from build123d import *

# Parameters (mm, degrees)
F0_R     = 6.35
F1_DEPTH = 25.4
F3_DEPTH = 12.7
F4_W     = 6.35
F4_H     = 114.3
F5_DEPTH = 25.4


with BuildPart() as f1:
    # F0 (on Front) → F1 (new body)
    with BuildSketch(Plane.XZ):
        with Locations((3.9284797385, 25.3006741405)):
            Circle(F0_R)
    extrude(amount=F1_DEPTH)



with BuildPart() as f1b:
    # F0 (on Front) → F1, piece 2 (new body)
    with BuildSketch(Plane.XZ):
        with Locations((3.9284797385, -177.8993258595)):
            Circle(F0_R)
    extrude(amount=F1_DEPTH)


with BuildPart() as f1_1:
    add(f1.part)

    add(f1b.part)  # F3 merges F1b
    # F2 (on face) → F3 (join)
    with BuildSketch(Plane.XZ.offset(25.4)):
        with BuildLine():
            ThreePointArc((3.9284797385, 57.0506741405), (-18.5221605641, 47.7513144431), (-27.8215202615, 25.3006741405))
            Line((-27.8215202615, 25.3006741405), (-27.8215202615, -177.8993258595))
            ThreePointArc((-27.8215202615, -177.8993258595), (-18.5221605641, -200.3499661622), (3.9284797385, -209.6493258595))
            ThreePointArc((3.9284797385, -209.6493258595), (26.3791200412, -200.3499661622), (35.6784797385, -177.8993258595))
            Line((35.6784797385, -177.8993258595), (35.6784797385, 25.3006741405))
            ThreePointArc((35.6784797385, 25.3006741405), (26.3791200412, 47.7513144431), (3.9284797385, 57.0506741405))
        make_face()
        with BuildLine():
            ThreePointArc((3.9284797385, -6.4493258595), (8.4186077991, -8.309197799), (10.2784797385, -12.7993258595))
            Line((10.2784797385, -12.7993258595), (10.2784797385, -139.7993258595))
            ThreePointArc((10.2784797385, -139.7993258595), (8.4186077991, -144.2894539201), (3.9284797385, -146.1493258595))
            ThreePointArc((3.9284797385, -146.1493258595), (-0.561648322, -144.2894539201), (-2.4215202615, -139.7993258595))
            Line((-2.4215202615, -139.7993258595), (-2.4215202615, -12.7993258595))
            ThreePointArc((-2.4215202615, -12.7993258595), (-0.561648322, -8.309197799), (3.9284797385, -6.4493258595))
        make_face(mode=Mode.SUBTRACT)
    extrude(amount=F3_DEPTH)

    # F4 (on face) → F5 (join)
    with BuildSketch(Plane(origin=(0, -25.4, 0), x_dir=(-1, 0, 0), z_dir=(0, 1, 0))):
        with Locations((5.5965202615, -76.2993258595)):
            Rectangle(F4_W, F4_H)
        with Locations((-13.4534797385, -76.2993258595)):
            Rectangle(F4_W, F4_H)
    extrude(amount=F5_DEPTH)


solid = f1_1.part
The model under review builds one solid part; all positions refer to its coordinate system, in mm. A direction names the side the tool comes from. Round coordinates to 2 decimals unless told otherwise and drop trailing zeros. Order: outer loops, then holes, each group sorted by start corner. A loop starts at its lowest first (then second) coordinate and runs counter-clockwise, first axis right, second up. Notation, with made-up numbers: (19, -2) -> (78, -2) arc R27 cw to (78, 20) -> close; hole circle Ø11 at (5, -35). An arc over 180 degrees is marked (long way). Return JSON: item names as keys, results as strings.
1. Take a section at B-B (y = -34.5). Write out the cut boundary in (x, z), then the cut area to 3 significant figures.
Answer block:
{"outline": "(-27.82, -177.9) arc R31.75 ccw to (35.68, -177.9) -> (35.68, 25.3) arc R31.75 ccw to (-27.82, 25.3) -> close; hole (-2.42, -139.8) arc R6.35 ccw to (10.28, -139.8) -> (10.28, -12.8) arc R6.35 ccw to (-2.42, -12.8) -> close", "area": "14,300 mm²"}
2. Take a section at C-C (y = -9.5). Write out the cut boundary in (x, z).
Answer block:
{"outline": "(-8.77, -133.45) -> (-2.42, -133.45) -> (-2.42, -19.15) -> (-8.77, -19.15) -> close; circle Ø12.7 at (3.93, -177.9); circle Ø12.7 at (3.93, 25.3); (10.28, -133.45) -> (16.63, -133.45) -> (16.63, -19.15) -> (10.28, -19.15) -> close"}
3. The part is to be moulded in two halves that separate along X. For faces 6 (the face through (11, -38.1, -74)), 7 (the face through (-8.772, -13, -77)), 8 (the face through (10.278, -19, -75)), say which applies: +X half, -X half, draft (parallel to the pull), parting line (faces both ways), or undercut.
Answer block:
{"face 6": "draft", "face 7": "-X half", "face 8": "undercut"}
4. Take a section at A-A (z = -37.5). Write out the cut boundary in (x, y), then the cut area to 3 significant figures.
Answer block:
{"outline": "(-27.82, -38.1) -> (-2.42, -38.1) -> (-2.42, 0) -> (-8.77, 0) -> (-8.77, -25.4) -> (-27.82, -25.4) -> close; (10.28, -38.1) -> (35.68, -38.1) -> (35.68, -25.4) -> (16.63, -25.4) -> (16.63, 0) -> (10.28, 0) -> close", "area": "968 mm²"}
5. Take a section at D-D (z = 6.5). Write out the cut boundary in (x, y).
Answer block:
{"outline": "(-27.82, -38.1) -> (35.68, -38.1) -> (35.68, -25.4) -> (-27.82, -25.4) -> close"}
6. Insertion check: P1, Ø6, axis at x = -11, z = -47, coming from the +Y side; P2, Ø1.9, axis at x = -6.5, y = -19, coming from the -Z side; P3, Ø6, axis at x = 17, y = -10.5, coming from the +Z side; P4, Ø3, axis at x = 7, y = -14, coming from the -Z side. Each pin has a flat end and moves straight along its axis. Give the tip position at first contact, or say it passes through.
Answer block:
{"P1": "stops at y = 0", "P2": "stops at z = -133.45", "P3": "stops at z = -19.15", "P4": "stops at z = -184.05"}
7. For faces 1 (the face through (-2.422, -19, -77)), 2 (the face through (13, -13, -133.449)), 3 (the face through (-6, -13, -19.149)), 4 (the face through (3.102, -12.522, 31.597)), 5 (the face through (16.628, -13, -77)), list the 3-axis set-ups (+Z, -Z, +X, -X, +Y, -Y) from which the entire face can be reached by the end or side of a thin tool; tool diameter is ignored.
Answer block:
{"face 1": "+Y, -Y", "face 2": "-Z, +X, -X, +Y", "face 3": "+Z, +X, -X, +Y", "face 4": "+Y", "face 5": "+Z, -Z, +X, +Y"}
8. For L1, parallel to X at y = -24, z = -127.5; L2, parallel to X at y = -33.5, z = -17; L3, parallel to Z at x = -6, y = -5, list the stretches that pass through material, from the lowest coordinate up. Write a range as [from, to].
Answer block:
{"L1": "x = [-8.77, -2.42], [10.28, 16.63]", "L2": "x = [-27.82, -2.42], [10.28, 35.68]", "L3": "z = [-133.45, -19.15]"}
